CAD build for the part. Positions are in the model's coordinates, mm. A direction names the side the tool comes from. Give positions to 0.01 mm unless a question says otherwise; leave off trailing zeros. Loops run counter-clockwise (first coordinate to the right, second up) from the corner with the lowest first, then second, coordinate; pieces in that order, holes last. Notation, with made-up numbers: M 8,89 L 55,89 A28 ccw 55,124 Z; hole C 58,62 d1. An arc over 180 degrees is marked long. Answer as CSV lines item,"result".
from build123d import *

# Parameters (mm, degrees)
SKETCH1_R           = 1.7
SKETCH1_R_2         = 13.5
SKETCH1_R_3         = 3
SKETCH1_R_4         = 11.05
BOSS_EXTRUDE1_DEPTH = 2.54


with BuildPart() as part:
    # Sketch1 → Boss-Extrude1 (new body)
    with BuildSketch(Plane(origin=(0, 0, 0), x_dir=(1, 0, 0), z_dir=(0, 1, 0))):
        with BuildLine():
            ThreePointArc((0, 49), (22.160822156, 43.702379356), (39.529822722, 28.955018831))
            Line((39.529822722, 28.955018831), (48, 28.955018831))
            ThreePointArc((48, 28.955018831), (75.385415079, 0), (48, -28.955018831))
            Line((48, -28.955018831), (39.529822722, -28.955018831))
            ThreePointArc((39.529822722, -28.955018831), (22.160822156, -43.702379356), (0, -49))
            ThreePointArc((0, -49), (-49, 0), (0, 49))
        make_face()
        with Locations(Location((38.100505063, -9.899494937, 0), (0, 0, 270))):
            Circle(SKETCH1_R, mode=Mode.SUBTRACT)
        with Locations(Location((57.899494937, -9.899494937, 0), (0, 0, 270))):
            Circle(SKETCH1_R, mode=Mode.SUBTRACT)
        with Locations(Location((57.899494937, 9.899494937, 0), (0, 0, 270))):
            Circle(SKETCH1_R, mode=Mode.SUBTRACT)
        with Locations(Location((38.100505063, 9.899494937, 0), (0, 0, 270))):
            Circle(SKETCH1_R, mode=Mode.SUBTRACT)
        with Locations(Location((0, 0, 0), (0, 0, 270))):
            Circle(SKETCH1_R_2, mode=Mode.SUBTRACT)
        with Locations(Location((-12.572358569, -12.572358569, 0), (0, 0, 270))):
            Circle(SKETCH1_R_3, mode=Mode.SUBTRACT)
        with Locations(Location((12.572358569, -12.572358569, 0), (0, 0, 270))):
            Circle(SKETCH1_R_3, mode=Mode.SUBTRACT)
        with Locations(Location((12.572358569, 12.572358569, 0), (0, 0, 270))):
            Circle(SKETCH1_R_3, mode=Mode.SUBTRACT)
        with Locations(Location((-12.572358569, 12.572358569, 0), (0, 0, 270))):
            Circle(SKETCH1_R_3, mode=Mode.SUBTRACT)
        with Locations(Location((48, 0, 0), (0, 0, 270))):
            Circle(SKETCH1_R_4, mode=Mode.SUBTRACT)
    extrude(amount=BOSS_EXTRUDE1_DEPTH)


solid = part.part
1) Band-saw the part on C-C on y = 0.8. Give the number of separate pieces and of enclosed holes in the cut face, and give its area (3 significant figures).
Answer below:
separate pieces,"1"
enclosed holes,"10"
area,"7,780 mm^2"
2) Which spindle directions (+Z, -Z, +X, -X, +Y, -Y) get a long thin tool onto all of the face, cutting with end or side? Do faces 5 (the face through (44, 1, -28.955)), 6 (the face through (15.547, 1.252, -12.963)), 7 (the face through (44, 1, 28.955)). Say none if no direction does.
Answer below:
face 5,"-Z, +X, +Y, -Y"
face 6,"+Y, -Y"
face 7,"+Z, +X, +Y, -Y"
3) Mould opens along Z. For faces 1 (the face through (-14.4, 1.25, -14.95)), 2 (the face through (14, 2.54, -1)), 3 (the face through (39.534, 1.252, -8.986)), 4 (the face through (75.38, 1.25, -0.62)) say: +Z half, -Z half, draft (parallel to the pull), parting line (faces both ways), or undercut.
Answer below:
face 1,"undercut"
face 2,"draft"
face 3,"undercut"
face 4,"parting line"
4) Band-saw the part on A-A on z = 0. Give the cut face in (x, y).
Answer below:
outline,"M -49,0 L -13.5,0 L -13.5,2.54 L -49,2.54 Z; M 13.5,0 L 36.95,0 L 36.95,2.54 L 13.5,2.54 Z; M 59.05,0 L 75.39,0 L 75.39,2.54 L 59.05,2.54 Z"
5) Band-saw the part on B-B on x = 3. Give the cut face in (y, z).
Answer below:
outline,"M 0,-48.91 L 2.54,-48.91 L 2.54,-13.16 L 0,-13.16 Z; M 0,13.16 L 2.54,13.16 L 2.54,48.91 L 0,48.91 Z"
6) Flat gauge pins, fed straight in: pin 1 (0.8 mm diameter, centred on x = 44, y = 1.5, fed in from -Z) (3 decimals); pin 2 (1.3 mm diameter, centred on x = 44.5, y = 1, fed in from +Z) (3 decimals); pin 3 (1 mm diameter, centred on y = 1, z = -25.5, fed in from +X). Where does each tip first touch, or does it go through?
Answer below:
pin 1,"stops at z = -28.955"
pin 2,"stops at z = 28.955"
pin 3,"stops at x = 61.08"
7) Band-saw the part on D-D on x = -22. Give the cut face in (y, z), and give its area (3 significant figures).
Answer below:
outline,"M 0,-43.78 L 2.54,-43.78 L 2.54,43.78 L 0,43.78 Z"
area,"222 mm^2"
8) Drill centre lines: line 1 (X direction, y = 0.7, z = -5); line 2 (X direction, y = 1.15, z = -14); line 3 (X direction, y = 1.85, z = -9). Where is each one in solid material? Low to high. Write a range as from..to.
Answer below:
line 1,"x = -48.74..-12.54, 12.54..38.15, 57.85..74.95"
line 2,"x = -46.96..-15.21, -9.93..9.93, 15.21..71.78"
line 3,"x = -48.17..-10.06, 10.06..36.66, 39.54..41.59, 54.41..56.46, 59.34..73.95"
